Answer from the drawing. Dimensions are ordinates in mm from the lowest x, y and z of the part. A direction names the side the tool comes from. Coordinates: 2 decimals unless noted, no trailing zeros. Write each loop counter-clockwise with the first axis right and the second up, starting at its lowest first coordinate (ties: lowest second). Pieces come first, ordered by that corner, then holes. Notation, with made-up numbers: (60.25, 14.5) -> (88.25, 14.5) arc R15 cw to (88.25, 32.5) -> close; hole circle Ø1 at (19.5, 56.5). An arc over 180 degrees is marked (long way). One line per item, written item: value. Start each with the question number.
1. Find section C-C, the plane x = 4. Write down the section's boundary in (y, z), and give its area (3 significant figures).
2. Find section A-A, the plane z = 32. Write down the section's boundary in (x, y).
3. Find section B-B, the plane y = 24. Write down the section's boundary in (x, z).
4. Consider line 1 along Y through (x, z) = (21.15, 32); line 2 along Z through (x, y) = (15.5, 11); line 3 along X through (y, z) = (23.5, 30.5). Determine where each line is inside the solid, lowest interval first.
5. Given P1, Ø6, axis at x = 16, z = 20.5, coming from the -Y side; P2, Ø4, axis at y = 24, z = 32, coming from the -X side; P3, Ø6, axis at x = 4, y = 5, coming from the +Z side; P4, Ø3.5, axis at x = 4, y = 4, coming from the +Z side, each flat-ended and moving along its own axis, determine where each tip first touches the part or whether it passes through.
6. Find section D-D, the plane z = 21.5. Write down the section's boundary in (x, y), and give its area (3 significant figures).
7. For the marked faces 1 and 2, determine the directions among +Z, -Z, +X, -X, +Y, -Y from which every point of the face is accessible in a straight line to the end or side of a thin tool.
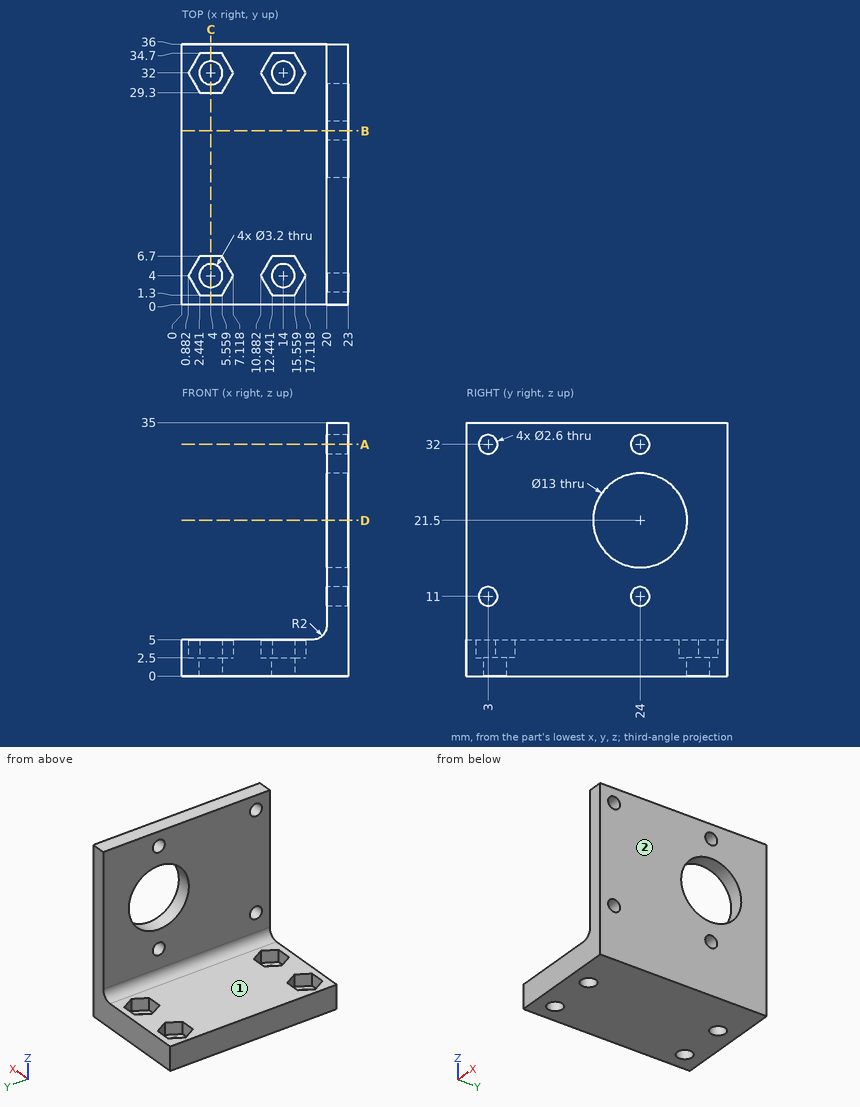
Answer block:
1. outline: (0, 0) -> (2.4, 0) -> (2.4, 2.5) -> (1.3, 2.5) -> (1.3, 5) -> (0, 5) -> close; (5.6, 0) -> (30.4, 0) -> (30.4, 2.5) -> (29.3, 2.5) -> (29.3, 5) -> (6.7, 5) -> (6.7, 2.5) -> (5.6, 2.5) -> close; (33.6, 0) -> (36, 0) -> (36, 5) -> (34.7, 5) -> (34.7, 2.5) -> (33.6, 2.5) -> close
1. area: 137 mm2
2. outline: (20, 0) -> (23, 0) -> (23, 1.7) -> (20, 1.7) -> close; (20, 4.3) -> (23, 4.3) -> (23, 22.7) -> (20, 22.7) -> close; (20, 25.3) -> (23, 25.3) -> (23, 36) -> (20, 36) -> close
3. outline: (0, 0) -> (23, 0) -> (23, 9.7) -> (20, 9.7) -> (20, 7) arc R2 cw to (18, 5) -> (0, 5) -> close; (20, 12.3) -> (23, 12.3) -> (23, 15) -> (20, 15) -> close; (20, 28) -> (23, 28) -> (23, 30.7) -> (20, 30.7) -> close; (20, 33.3) -> (23, 33.3) -> (23, 35) -> (20, 35) -> close
4. line 1: y = 0 to 1.7, 4.3 to 22.7, 25.3 to 36
4. line 2: z = 0 to 5
4. line 3: x = 20 to 23
5. P1: passes through
5. P2: stops at x = 20
5. P3: stops at z = 5
5. P4: stops at z = 2.5
6. outline: (20, 0) -> (23, 0) -> (23, 17.5) -> (20, 17.5) -> close; (20, 30.5) -> (23, 30.5) -> (23, 36) -> (20, 36) -> close
6. area: 69.0 mm2
7. face 1: +Z, -X, +Y, -Y
7. face 2: +Z, -Z, +X, +Y, -Y
